Verification items for the finished model (mm, model axes). A direction names the side the tool comes from. Round coordinates to 2 decimals unless told otherwise and drop trailing zeros. Loops run counter-clockwise (first coordinate to the right, second up) from the corner with the lowest first, then second, coordinate; pieces in that order, holes last. Notation, with made-up numbers: M 16.25,61.25 L 65.25,61.25 A13 cw 65.25,82.25 Z; hole C 88.25,-4.5 d6. An arc over 180 degrees is marked long. Answer as CSV lines item,"result".
```python
from build123d import *

# Parameters (mm, degrees)
BOSS_EXTRUDE1_DEPTH = 2.5
SKETCH2_R           = 1.7
CUT_EXTRUDE1_DEPTH  = 1.5
FILLET1_R           = 1.5


with BuildPart() as part:
    # Sketch1 → Boss-Extrude1 (new body)
    with BuildSketch(Plane.XY):
        Polygon((-7.56419618, 12.7), (-7.56419618, 9.2), (6.18580382, 0), (6.18580382, 12.7), align=None)
    extrude(amount=BOSS_EXTRUDE1_DEPTH)

    # Sketch2 → Cut-Extrude1 (cut)
    with BuildSketch(Plane.XY.offset(2.5)):
        with Locations((-4.31419618, 9.2)):
            Circle(SKETCH2_R)
    extrude(amount=-CUT_EXTRUDE1_DEPTH, mode=Mode.SUBTRACT)

    # Mirror2: part across plane


with BuildPart() as part_1:
    add(part.part)
    add(part.part.mirror(Plane(origin=(6.18580382, 0, 2.5), x_dir=(0, 0, 1), z_dir=(-1, 0, 0))))

    # Fillet1
    fillet1_edges = [part_1.edges().sort_by_distance(p)[0] for p in [
        (19.93580382, 12.7, 1.25),
        (19.93580382, 9.2, 1.25),
        (6.18580382, 0, 1.25),
        (19.93580382, 10.95, 0),
        (13.06080382, 4.6, 0),
        (-0.68919618, 4.6, 0),
        (-7.56419618, 10.95, 0),
        (6.18580382, 12.7, 0),
        (-7.56419618, 9.2, 1.25),
        (-7.56419618, 12.7, 1.25),
    ]]
    fillet(fillet1_edges, radius=FILLET1_R)


solid = part_1.part
```
1) Draft check along X on faces 1 (the cylindrical face through (18.384, 9.275, 1.76)), 2 (the cylindrical face through (-7.136, 10.592, 0.451)), 3 (the flat face through (6, 8, 0)). Enter one of: +X half, -X half, draft (parallel to the pull), parting line (faces both ways), or undercut.
Here are the results:
face 1,"undercut"
face 2,"-X half"
face 3,"draft"
2) Set-up check for faces 4 (the flat face through (-0.859, 4.714, 1.993)), 5 (the cylindrical face through (-4.536, 10.886, 1.76)): record each of +Z, -Z, +X, -X, +Y, -Y from which the full face is reachable in a straight line by a thin tool's end or side.
Here are the results:
face 4,"+Z, -Z, -X, -Y"
face 5,"+Z"
3) Section check A-A (z = 2.1). Record the cut outline in (x, y), plus the area to 3 significant figures.
Here are the results:
outline,"M -7.56,10 A1.5 ccw -6.9,8.75 L 5.35,0.56 A1.5 ccw 7.02,0.56 L 19.27,8.75 A1.5 ccw 19.94,10 L 19.94,11.2 A1.5 ccw 18.44,12.7 L -6.06,12.7 A1.5 ccw -7.56,11.2 Z; hole C -4.31,9.2 d3.4; hole C 16.69,9.2 d3.4"
area,"203 mm^2"
4) Section check B-B (z = 0.65). Record the cut outline in (x, y), plus the area to 3 significant figures.
Here are the results:
outline,"M -7.3,10 A1.24 ccw -6.75,8.97 L 5.5,0.78 A1.24 ccw 6.87,0.78 L 19.12,8.97 A1.24 ccw 19.67,10 L 19.67,11.2 A1.24 ccw 18.44,12.44 L -6.06,12.44 A1.24 ccw -7.3,11.2 Z"
area,"204 mm^2"
5) Go/stop test with flat-tipped pins: pin 1 (2 mm diameter, centred on x = -4.31, y = 9.2, fed in from +Z); pin 2 (2 mm diameter, centred on x = -3.5, y = 3, fed in from -Z). Record where each tip stops, or that it passes through.
Here are the results:
pin 1,"stops at z = 1"
pin 2,"passes through"
6) Material ranges on probe 1 along X at (y, z) = (8, 2.2); probe 2 along Y at (x, z) = (-3, 1.05); probe 3 along X at (y, z) = (3.25, 0.65), recorded low to high.
Here are the results:
probe 1,"x = -5.77 to -5.52, -3.11 to 15.48, 17.89 to 18.14"
probe 2,"y = 6.23 to 8.12, 10.28 to 12.63"
probe 3,"x = 1.8 to 10.57"
